```python
from build123d import *

# Parameters (mm, degrees)
SKETCH1_W              = 7.5
SKETCH1_H              = 5.6
EXTRUDE1_DEPTH         = 6.6
CUT_EXTRUDE1_DEPTH     = 6.6
SKETCH3_W              = 6
SKETCH3_H              = 4.1
CUT_EXTRUDE2_DEPTH     = 5.25
SKETCH5_W              = 1.27
SKETCH5_H              = 3
CUT_EXTRUDE3_DEPTH     = 8.5
CUT_EXTRUDE4_DEPTH     = 1.2
FILLET1_R              = 0.5
EXTRUDE2_DEPTH         = 6.3
EXTRUDE2_DEPTH_BACK    = 2
CHAMFER1_SIZE          = 0.5
CHAMFER1_SIZE2         = 0.08816349
CHAMFER1_PART_2_SIZE   = 0.5
CHAMFER1_PART_2_SIZE2  = 0.08816349
CHAMFER1_PART_3_SIZE   = 0.5
CHAMFER1_PART_3_SIZE2  = 0.08816349
CHAMFER1_PART_4_SIZE   = 0.5
CHAMFER1_PART_4_SIZE2  = 0.08816349
CHAMFER1_PART_5_SIZE   = 0.5
CHAMFER1_PART_5_SIZE2  = 0.08816349
CHAMFER1_PART_6_SIZE   = 0.5
CHAMFER1_PART_6_SIZE2  = 0.08816349
CHAMFER1_PART_7_SIZE   = 0.5
CHAMFER1_PART_7_SIZE2  = 0.08816349
CHAMFER1_PART_8_SIZE   = 0.5
CHAMFER1_PART_8_SIZE2  = 0.08816349
CHAMFER1_PART_9_SIZE   = 0.5
CHAMFER1_PART_9_SIZE2  = 0.08816349
CHAMFER1_PART_10_SIZE  = 0.5
CHAMFER1_PART_10_SIZE2 = 0.08816349
CHAMFER1_PART_11_SIZE  = 0.5
CHAMFER1_PART_11_SIZE2 = 0.08816349
CHAMFER1_PART_12_SIZE  = 0.5
CHAMFER1_PART_12_SIZE2 = 0.08816349
CHAMFER1_PART_13_SIZE  = 0.5
CHAMFER1_PART_13_SIZE2 = 0.08816349
CHAMFER1_PART_14_SIZE  = 0.5
CHAMFER1_PART_14_SIZE2 = 0.08816349
CHAMFER1_PART_15_SIZE  = 0.5
CHAMFER1_PART_15_SIZE2 = 0.08816349
CHAMFER1_PART_16_SIZE  = 0.5
CHAMFER1_PART_16_SIZE2 = 0.08816349


with BuildPart() as part:
    # Sketch1 → Extrude1 (new body)
    with BuildSketch(Plane(origin=(0, 0, 0), x_dir=(1, 0, 0), z_dir=(0, 1, 0))):
        Rectangle(SKETCH1_W, SKETCH1_H)
    extrude(amount=EXTRUDE1_DEPTH)

    # Sketch2 → Cut-Extrude1 (cut, through all)
    with BuildSketch(Plane.XY.offset(2.8)):
        Polygon((-1.995, 0.65), (-0.545, 0.65), (-0.545, 0), (-1.27, 0), (-1.995, 0), align=None)
        Polygon((0.545, 0.65), (1.995, 0.65), (1.995, 0), (1.27, 0), (0.545, 0), align=None)
    extrude(amount=-CUT_EXTRUDE1_DEPTH, mode=Mode.SUBTRACT)

    # Sketch3 → Cut-Extrude2 (cut)
    with BuildSketch(Plane(origin=(0, 6.6, 0), x_dir=(-1, 0, 0), z_dir=(0, 1, 0))):
        Rectangle(SKETCH3_W, SKETCH3_H)
    extrude(amount=-CUT_EXTRUDE2_DEPTH, mode=Mode.SUBTRACT)

    # Sketch5 → Cut-Extrude3 (cut, through all)
    with BuildSketch(Plane.ZY.offset(3.75)):
        with Locations((-1.415, 5.1)):
            Rectangle(SKETCH5_W, SKETCH5_H)
    extrude(amount=-CUT_EXTRUDE3_DEPTH, mode=Mode.SUBTRACT)

    # Sketch6 → Cut-Extrude4 (cut)
    with BuildSketch(Plane(origin=(0, 0, -2.8), x_dir=(-1, 0, 0), z_dir=(0, 0, -1))):
        Polygon((-1.75, 6.6), (1.75, 6.6), (1.299695014, 5.694073356), (1.75, 5.606485511), (1.75, 2.666508092), (-1.75, 2.666508092), (-1.75, 5.606485511), (-1.299695014, 5.694073356), align=None)
    extrude(amount=-CUT_EXTRUDE4_DEPTH, mode=Mode.SUBTRACT)

    # Fillet1
    fillet1_edges = [part.edges().sort_by_distance(p)[0] for p in [
        (-1.75, 2.666508092, -2.425),
        (1.75, 2.666508092, -2.425),
    ]]
    fillet(fillet1_edges, radius=FILLET1_R)

    # Sketch7 → Extrude2 (add, two sides)
    with BuildSketch(Plane(origin=(0, 0, 0), x_dir=(1, 0, 0), z_dir=(0, 1, 0))) as extrude2_sk:
        Polygon((-1.27, -0.040243902), (-0.945, -0.040243902), (-0.945, 0.609756098), (-1.595, 0.609756098), (-1.595, -0.040243902), align=None)
        Polygon((1.27, -0.040243902), (0.945, -0.040243902), (0.945, 0.609756098), (1.595, 0.609756098), (1.595, -0.040243902), align=None)
    extrude(amount=EXTRUDE2_DEPTH)
    extrude(extrude2_sk.sketch, amount=-EXTRUDE2_DEPTH_BACK)

    # Chamfer1
    chamfer1_edges = [part.edges().sort_by_distance(p)[0] for p in [
        (-1.595, -2, -0.284756098),
    ]]
    chamfer1_side = [part.faces().sort_by_distance(p)[0] for p in [
        (-1.595, -0.675, -0.284756098),
    ]]
    chamfer(chamfer1_edges, length=CHAMFER1_SIZE, length2=CHAMFER1_SIZE2, reference=chamfer1_side[0])

    # Chamfer1 part 2
    chamfer1_part_2_edges = [part.edges().sort_by_distance(p)[0] for p in [
        (-1.27, -2, 0.040243902),
    ]]
    chamfer1_part_2_side = [part.faces().sort_by_distance(p)[0] for p in [
        (-1.27, -0.675, 0.040243902),
    ]]
    chamfer(chamfer1_part_2_edges, length=CHAMFER1_PART_2_SIZE, length2=CHAMFER1_PART_2_SIZE2, reference=chamfer1_part_2_side[0])

    # Chamfer1 part 3
    chamfer1_part_3_edges = [part.edges().sort_by_distance(p)[0] for p in [
        (-0.945, -2, -0.284756098),
    ]]
    chamfer1_part_3_side = [part.faces().sort_by_distance(p)[0] for p in [
        (-0.945, -0.675, -0.284756098),
    ]]
    chamfer(chamfer1_part_3_edges, length=CHAMFER1_PART_3_SIZE, length2=CHAMFER1_PART_3_SIZE2, reference=chamfer1_part_3_side[0])

    # Chamfer1 part 4
    chamfer1_part_4_edges = [part.edges().sort_by_distance(p)[0] for p in [
        (-1.27, -2, -0.609756098),
    ]]
    chamfer1_part_4_side = [part.faces().sort_by_distance(p)[0] for p in [
        (-1.27, -0.675, -0.609756098),
    ]]
    chamfer(chamfer1_part_4_edges, length=CHAMFER1_PART_4_SIZE, length2=CHAMFER1_PART_4_SIZE2, reference=chamfer1_part_4_side[0])

    # Chamfer1 part 5
    chamfer1_part_5_edges = [part.edges().sort_by_distance(p)[0] for p in [
        (-1.27, 6.3, -0.609756098),
    ]]
    chamfer1_part_5_side = [part.faces().sort_by_distance(p)[0] for p in [
        (-1.27, 3.825, -0.609756098),
    ]]
    chamfer(chamfer1_part_5_edges, length=CHAMFER1_PART_5_SIZE, length2=CHAMFER1_PART_5_SIZE2, reference=chamfer1_part_5_side[0])

    # Chamfer1 part 6
    chamfer1_part_6_edges = [part.edges().sort_by_distance(p)[0] for p in [
        (-1.595, 6.3, -0.284756098),
    ]]
    chamfer1_part_6_side = [part.faces().sort_by_distance(p)[0] for p in [
        (-1.595, 3.825, -0.284756098),
    ]]
    chamfer(chamfer1_part_6_edges, length=CHAMFER1_PART_6_SIZE, length2=CHAMFER1_PART_6_SIZE2, reference=chamfer1_part_6_side[0])

    # Chamfer1 part 7
    chamfer1_part_7_edges = [part.edges().sort_by_distance(p)[0] for p in [
        (-1.27, 6.3, 0.040243902),
    ]]
    chamfer1_part_7_side = [part.faces().sort_by_distance(p)[0] for p in [
        (-1.27, 3.825, 0.040243902),
    ]]
    chamfer(chamfer1_part_7_edges, length=CHAMFER1_PART_7_SIZE, length2=CHAMFER1_PART_7_SIZE2, reference=chamfer1_part_7_side[0])

    # Chamfer1 part 8
    chamfer1_part_8_edges = [part.edges().sort_by_distance(p)[0] for p in [
        (-0.945, 6.3, -0.284756098),
    ]]
    chamfer1_part_8_side = [part.faces().sort_by_distance(p)[0] for p in [
        (-0.945, 3.825, -0.284756098),
    ]]
    chamfer(chamfer1_part_8_edges, length=CHAMFER1_PART_8_SIZE, length2=CHAMFER1_PART_8_SIZE2, reference=chamfer1_part_8_side[0])

    # Chamfer1 part 9
    chamfer1_part_9_edges = [part.edges().sort_by_distance(p)[0] for p in [
        (1.595, -2, -0.284756098),
    ]]
    chamfer1_part_9_side = [part.faces().sort_by_distance(p)[0] for p in [
        (1.595, -0.675, -0.284756098),
    ]]
    chamfer(chamfer1_part_9_edges, length=CHAMFER1_PART_9_SIZE, length2=CHAMFER1_PART_9_SIZE2, reference=chamfer1_part_9_side[0])

    # Chamfer1 part 10
    chamfer1_part_10_edges = [part.edges().sort_by_distance(p)[0] for p in [
        (1.27, -2, -0.609756098),
    ]]
    chamfer1_part_10_side = [part.faces().sort_by_distance(p)[0] for p in [
        (1.27, -0.675, -0.609756098),
    ]]
    chamfer(chamfer1_part_10_edges, length=CHAMFER1_PART_10_SIZE, length2=CHAMFER1_PART_10_SIZE2, reference=chamfer1_part_10_side[0])

    # Chamfer1 part 11
    chamfer1_part_11_edges = [part.edges().sort_by_distance(p)[0] for p in [
        (0.945, -2, -0.284756098),
    ]]
    chamfer1_part_11_side = [part.faces().sort_by_distance(p)[0] for p in [
        (0.945, -0.675, -0.284756098),
    ]]
    chamfer(chamfer1_part_11_edges, length=CHAMFER1_PART_11_SIZE, length2=CHAMFER1_PART_11_SIZE2, reference=chamfer1_part_11_side[0])

    # Chamfer1 part 12
    chamfer1_part_12_edges = [part.edges().sort_by_distance(p)[0] for p in [
        (1.27, -2, 0.040243902),
    ]]
    chamfer1_part_12_side = [part.faces().sort_by_distance(p)[0] for p in [
        (1.27, -0.675, 0.040243902),
    ]]
    chamfer(chamfer1_part_12_edges, length=CHAMFER1_PART_12_SIZE, length2=CHAMFER1_PART_12_SIZE2, reference=chamfer1_part_12_side[0])

    # Chamfer1 part 13
    chamfer1_part_13_edges = [part.edges().sort_by_distance(p)[0] for p in [
        (1.27, 6.3, 0.040243902),
    ]]
    chamfer1_part_13_side = [part.faces().sort_by_distance(p)[0] for p in [
        (1.27, 3.825, 0.040243902),
    ]]
    chamfer(chamfer1_part_13_edges, length=CHAMFER1_PART_13_SIZE, length2=CHAMFER1_PART_13_SIZE2, reference=chamfer1_part_13_side[0])

    # Chamfer1 part 14
    chamfer1_part_14_edges = [part.edges().sort_by_distance(p)[0] for p in [
        (1.595, 6.3, -0.284756098),
    ]]
    chamfer1_part_14_side = [part.faces().sort_by_distance(p)[0] for p in [
        (1.595, 3.825, -0.284756098),
    ]]
    chamfer(chamfer1_part_14_edges, length=CHAMFER1_PART_14_SIZE, length2=CHAMFER1_PART_14_SIZE2, reference=chamfer1_part_14_side[0])

    # Chamfer1 part 15
    chamfer1_part_15_edges = [part.edges().sort_by_distance(p)[0] for p in [
        (1.27, 6.3, -0.609756098),
    ]]
    chamfer1_part_15_side = [part.faces().sort_by_distance(p)[0] for p in [
        (1.27, 3.825, -0.609756098),
    ]]
    chamfer(chamfer1_part_15_edges, length=CHAMFER1_PART_15_SIZE, length2=CHAMFER1_PART_15_SIZE2, reference=chamfer1_part_15_side[0])

    # Chamfer1 part 16
    chamfer1_part_16_edges = [part.edges().sort_by_distance(p)[0] for p in [
        (0.945, 6.3, -0.284756098),
    ]]
    chamfer1_part_16_side = [part.faces().sort_by_distance(p)[0] for p in [
        (0.945, 3.825, -0.284756098),
    ]]
    chamfer(chamfer1_part_16_edges, length=CHAMFER1_PART_16_SIZE, length2=CHAMFER1_PART_16_SIZE2, reference=chamfer1_part_16_side[0])


solid = part.part
```
Geometry: final body of the model. Coordinates: model frame, mm. A direction names the side the tool comes from. Coordinates: 2 decimals unless noted, no trailing zeros. Order: outer loops, then holes, each group sorted by start corner. A loop starts at its lowest first (then second) coordinate and runs counter-clockwise, first axis right, second up.
Item 1: Section query D-D (x = -0.25). Output: boundary loops of the cut face in (y, z).
Answer:
outline: (0, -2.8) - (2.67, -2.8) - (2.67, -2.05) - (1.35, -2.05) - (1.35, 2.05) - (6.6, 2.05) - (6.6, 2.8) - (0, 2.8) - close
Item 2: Section query A-A (y = 1.75). Output: boundary loops of the cut face in (x, z) (3 decimals).
Answer:
outline: (-3.75, -2.8) - (3.75, -2.8) - (3.75, 2.8) - (-3.75, 2.8) - close; (-1.595, -0.61) - (-0.945, -0.61) - (-0.945, 0.04) - (-1.595, 0.04) - close; (0.945, -0.61) - (1.595, -0.61) - (1.595, 0.04) - (0.945, 0.04) - close; hole (-3, -2.05) - (3, -2.05) - (3, 2.05) - (-3, 2.05) - close
Item 3: Section query B-B (y = -1). Output: boundary loops of the cut face in (x, z) (3 decimals), then the cut area to 3 significant figures.
Answer:
outline: (-1.595, -0.61) - (-0.945, -0.61) - (-0.945, 0.04) - (-1.595, 0.04) - close; (0.945, -0.61) - (1.595, -0.61) - (1.595, 0.04) - (0.945, 0.04) - close
area: 0.845 mm2
Item 4: Contact query for flat-ended pins moving along their axis: P1, Ø0.5, axis at y = -0.5, z = 0, coming from the +X side (3 decimals); P2, Ø0.5, axis at x = -1, y = 3, coming from the -Z side; P3, Ø0.9, axis at x = 0, z = 1, coming from the -Y side. Output: stop coordinate, or through.
Answer:
P1: stops at x = 1.595
P2: stops at z = -0.61
P3: stops at y = 0
Item 5: Section query C-C (z = 0.35). Output: boundary loops of the cut face in (x, y) (3 decimals).
Answer:
outline: (-3.75, 0) - (-1.995, 0) - (-1.995, 0.65) - (-0.545, 0.65) - (-0.545, 0) - (0.545, 0) - (0.545, 0.65) - (1.995, 0.65) - (1.995, 0) - (3.75, 0) - (3.75, 6.6) - (3, 6.6) - (3, 1.35) - (-3, 1.35) - (-3, 6.6) - (-3.75, 6.6) - close
Item 6: Material intervals for line 1 along X through (y, z) = (2, -0.1) (3 decimals); line 2 along Z through (x, y) = (-1.25, 2.25); line 3 along Z through (x, y) = (1.25, 4.25), sorted ascending.
Answer:
line 1: x = -3.75 to -3, -1.595 to -0.945, 0.945 to 1.595, 3 to 3.75
line 2: z = -2.8 to -2.05, -0.61 to 0.04, 2.05 to 2.8
line 3: z = -0.61 to 0.04, 2.05 to 2.8
Item 7: Draft query along Z for faces 1 (the face through (0, 4, 2.05)), 2 (the face through (-3, 0, 0)), 3 (the face through (0, 2, -2.05)), 4 (the face through (0, 3, 2.8)). Return one class per face: released by +Z, released by -Z, zero draft, split by the parting line, or undercut.
Answer:
face 1: undercut
face 2: zero draft
face 3: undercut
face 4: released by +Z
Item 8: Access query for faces 5 (the face through (3.75, 3, 0)), 6 (the face through (-1.8, 0.65, 0)), 7 (the face through (0, 1.35, 0)). Directions: +Z, -Z, +X, -X, +Y, -Y. A direction counts if a zero-diameter tool reaches every point of the face in a straight line with its end or side. Return the directions, or none.
Answer:
face 5: +Z, -Z, +X, +Y, -Y
face 6: -Y
face 7: +Y
